Model file for the job. Use its own axes, mm. A direction names the side the tool comes from. Give positions to 0.01 mm unless a question says otherwise; leave off trailing zeros. Order: outer loops, then holes, each group sorted by start corner. A loop starts at its lowest first (then second) coordinate and runs counter-clockwise, first axis right, second up. Notation, with made-up numbers: (30, 34) - (76, 34) arc R17 ccw to (76, 53) - close; hole circle Ø1 at (63, 28). An arc over 180 degrees is marked (long way). Return JSON: item names as keys, results as strings. Group by question number.
from build123d import *

# Parameters (mm, degrees)
BOSS_EXTRUDE1_DEPTH = 20


with BuildPart() as part:
    # Sketch1 → Boss-Extrude1 (new body)
    with BuildSketch(Plane.XY):
        with BuildLine():
            Line((-25, 0.25), (-11.497282288, 0.25))
            Line((-11.497282288, 0.25), (-6.495190528, 0.25))
            ThreePointArc((-6.495190528, 0.25), (0, 6.5), (6.495190528, 0.25))
            Line((6.495190528, 0.25), (11.497282288, 0.25))
            Line((11.497282288, 0.25), (25, 0.25))
            Line((25, 0.25), (25, 5.25))
            Line((25, 5.25), (10.231690965, 5.25))
            ThreePointArc((10.231690965, 5.25), (0, 11.5), (-10.231690965, 5.25))
            Line((-10.231690965, 5.25), (-25, 5.25))
            Line((-25, 5.25), (-25, 0.25))
        make_face()
    extrude(amount=-BOSS_EXTRUDE1_DEPTH)


solid = part.part
(1) Slice it at D-D (y = 1). Give the cut face in (x, z).
(2) Slice it at C-C (x = 0). Give the cut face in (y, z).
(3) 3-axis set-ups, long thin cutter, end or side, ignore diameter. For faces 1 (the face through (0, 7, -20)), 2 (the face through (-18, 5.25, -10)), 3 (the face through (18, 5.25, -10)): which of +Z, -Z, +X, -X, +Y, -Y reach the whole face in a straight line?
(4) Drop flat-ended pins along their axis: pin 1 Ø6 at (x, z) = (3.5, -13.5) entering from +Y; pin 2 Ø4.5 at (x, z) = (-16.5, -10) entering from +Y; pin 3 Ø1 at (x, z) = (1, -11) entering from -Y. Give the stop position or say it passes through.
(5) Drill centre lines: L1, parallel to Y at x = 11, z = -12; L2, parallel to X at y = 6, z = -5.75; L3, parallel to X at y = 3.5, z = -15. Where is each one in solid material? Low to high.
(6) Pull direction X, two halves, no side cores. Call faces 4 (the face through (25, 3, -10)), 5 (the face through (-25, 3, -10)), 6 (the face through (-16, 0.25, -10)), 7 (the face through (-0.1, 6.5, -9.9)): released by +X, released by -X, zero draft, split by the parting line, or undercut.
(7) Slice it at A-A (y = 3). Give the cut face in (x, z).
Result set:
{
 "1": {"outline": "(-25, -20) - (-6.42, -20) - (-6.42, 0) - (-25, 0) - close; (6.42, -20) - (25, -20) - (25, 0) - (6.42, 0) - close"},
 "2": {"outline": "(6.5, -20) - (11.5, -20) - (11.5, 0) - (6.5, 0) - close"},
 "3": {"face 1": "-Z, +X, -X, +Y, -Y", "face 2": "+Z, -Z, -X, +Y", "face 3": "+Z, -Z, +X, +Y"},
 "4": {"pin 1": "stops at y = 11.49", "pin 2": "stops at y = 5.25", "pin 3": "stops at y = 6.32"},
 "5": {"L1": "y = 0.25 to 5.25", "L2": "x = -9.81 to -2.5, 2.5 to 9.81", "L3": "x = -25 to -5.48, 5.48 to 25"},
 "6": {"face 4": "released by +X", "face 5": "released by -X", "face 6": "zero draft", "face 7": "undercut"},
 "7": {"outline": "(-25, -20) - (-5.77, -20) - (-5.77, 0) - (-25, 0) - close; (5.77, -20) - (25, -20) - (25, 0) - (5.77, 0) - close"}
}
